```python
from build123d import *

# Parameters (mm, degrees)
SALIENTE_EXTRUIR1_DEPTH    = 25
CORTAR_EXTRUIR1_DEPTH      = 49.94129136
CORTAR_EXTRUIR1_DEPTH_BACK = 49.94129136
CROQUIS2_R                 = 8.375
SALIENTE_EXTRUIR2_DEPTH    = 3
SALIENTE_EXTRUIR3_DEPTH    = 3
CROQUIS5_R                 = 8.375
CORTAR_EXTRUIR2_DEPTH      = 83.95179323
CHAFL_N1_SIZE              = 10
CHAFL_N1_SIZE2             = 24.750868534
CROQUIS6_R                 = 1.625
SALIENTE_EXTRUIR4_DEPTH    = 3
CHAFL_N2_SIZE              = 3


with BuildPart() as part:
    # Croquis1 → Saliente-Extruir1 (new body)
    with BuildSketch(Plane(origin=(0, 0, 0), x_dir=(1, 0, 0), z_dir=(0, 1, 0))):
        Polygon((-26.5, 0), (-26.5, -30), (-29.5, -30), (-29.5, 3), (29.5, 3), (29.5, -30), (26.5, -30), (26.5, 0), align=None)
    extrude(amount=SALIENTE_EXTRUIR1_DEPTH)

    # Croquis2 → Cortar-Extruir1 (cut, two sides: drawn at the far end of the back side and taken through both)
    with BuildSketch(Plane.XY.offset(-CORTAR_EXTRUIR1_DEPTH_BACK)):
        with Locations((-12.925, 12.5)):
            Circle(CROQUIS2_R)
        with Locations(Location((12.925, 12.5, 0), (0, 0, 180))):
            Circle(CROQUIS2_R)
    extrude(amount=CORTAR_EXTRUIR1_DEPTH + CORTAR_EXTRUIR1_DEPTH_BACK, mode=Mode.SUBTRACT)

    # Croquis3 → Saliente-Extruir2 (add)
    with BuildSketch(Plane.ZY.offset(-26.5)):
        Polygon((0, 25), (30, 25), (30, 50), (0, 50), (-3, 50), (-3, 25), align=None)
    extrude(amount=-SALIENTE_EXTRUIR2_DEPTH)

    # Croquis4 → Saliente-Extruir3 (add)
    with BuildSketch(Plane.ZY.offset(29.5)):
        Polygon((0, 25), (30, 25), (30, 50), (0, 50), (-3, 50), (-3, 25), align=None)
    extrude(amount=-SALIENTE_EXTRUIR3_DEPTH)

    # Croquis5 → Cortar-Extruir2 (cut, through all)
    with BuildSketch(Plane.ZY.offset(29.5)):
        with Locations((17.5, 37.925)):
            Circle(CROQUIS5_R)
        with Locations((17.5, 12.075)):
            Circle(CROQUIS5_R)
    extrude(amount=-CORTAR_EXTRUIR2_DEPTH, mode=Mode.SUBTRACT)

    # Chaflán1
    chafl_n1_edges = [part.edges().sort_by_distance(p)[0] for p in [
        (26.5, 25, -1.5),
        (-26.5, 25, -1.5),
    ]]
    chafl_n1_side = [part.faces().sort_by_distance(p)[0] for p in [
        (0, 25, -1.5),
    ]]
    chamfer(chafl_n1_edges, length=CHAFL_N1_SIZE, length2=CHAFL_N1_SIZE2, reference=chafl_n1_side[0])

    # Croquis6 → Saliente-Extruir4 (add)
    # profile 1 of 2: a face of its own
    with BuildSketch(Plane.XY):
        Polygon((-29.5, 0), (-17.5, 0), (-12.5, 0), (-17.5, -5.001983983), (-17.5, -12), (-29.5, -12), align=None)
        with Locations((-23.5, -5.75)):
            Circle(CROQUIS6_R, mode=Mode.SUBTRACT)
    # profile 2 of 2: a face of its own
    with BuildSketch(Plane.XY):
        Polygon((12.5, 0), (17.5, 0), (29.5, 0), (29.5, -12), (17.5, -12), (17.5, -5.001983983), align=None)
        with Locations(Location((23.5, -5.75, 0), (0, 0, 180))):
            Circle(CROQUIS6_R, mode=Mode.SUBTRACT)
    extrude(amount=-SALIENTE_EXTRUIR4_DEPTH)

    # Chaflán2
    chafl_n2_edges = [part.edges().sort_by_distance(p)[0] for p in [
        (-29.5, -12, -1.5),
        (-17.5, -12, -1.5),
        (29.5, -12, -1.5),
        (17.5, -12, -1.5),
    ]]
    chamfer(chafl_n2_edges, length=CHAFL_N2_SIZE)


solid = part.part
```
Geometry check sheet. Reference: the model listing, model coordinates, mm. A direction names the side the tool comes from. Give positions to 0.01 mm unless a question says otherwise; leave off trailing zeros. Write each loop counter-clockwise with the first axis right and the second up, starting at its lowest first coordinate (ties: lowest second). Pieces come first, ordered by that corner, then holes.
1) Section check D-D, the plane z = 17.5. Record the boundary of the cut face in (x, y), and give its area (3 significant figures).
2) Release check for a two-part mould opening along Y. For faces 3 (the flat face through (-19, -10.5, -1.5)), 4 (the flat face through (26.5, 25, 13)), 5 (the cylindrical face through (-28.02, 3.9, 15.68)) record: pulls with the +Y half, pulls with the -Y half, needs draft (parallel to the pull), parting line crosses it, or undercut.
3) Section check A-A, the plane y = -5.75. Record the boundary of the cut face in (x, z) (3 decimals).
4) Access from +Z, -Z, +X, -X, +Y, -Y to the whole of each face (thin tool, end or side, straight path). Record for faces 1 (the flat face through (0, 0, -2)), 2 (the flat face through (-28, 25, 30)).
5) Gauge pin test, flat ends, axial feed: pin 1 (15 mm diameter, centred on y = 37.925, z = 17.5, fed in from -X); pin 2 (1.5 mm diameter, centred on x = -28.5, z = 9, fed in from -Y); pin 3 (19.5 mm diameter, centred on x = 12.925, y = 12.5, fed in from -Z); pin 4 (3.5 mm diameter, centred on x = 0, z = -1, fed in from +Y). Record the tip position at first contact, or that the pin passes through.
6) Section check B-B, the plane z = 3. Record the boundary of the cut face in (x, y).
7) Material ranges on L1, parallel to Y at x = 27, z = 17; L2, parallel to X at y = 27, z = 18; L3, parallel to Y at x = -27, z = 10.5, recorded low to high.
8) Section check C-C, the plane x = 23.5. Record the boundary of the cut face in (y, z) (3 decimals).
Computed:
1. outline: (-29.5, 0) - (-26.5, 0) - (-26.5, 3.7) - (-29.5, 3.7) - close; (-29.5, 20.45) - (-26.5, 20.45) - (-26.5, 29.55) - (-29.5, 29.55) - close; (-29.5, 46.3) - (-26.5, 46.3) - (-26.5, 50) - (-29.5, 50) - close; (26.5, 0) - (29.5, 0) - (29.5, 3.7) - (26.5, 3.7) - close; (26.5, 20.45) - (29.5, 20.45) - (29.5, 29.55) - (26.5, 29.55) - close; (26.5, 46.3) - (29.5, 46.3) - (29.5, 50) - (26.5, 50) - close
1. area: 99.0 mm2
2. face 3: pulls with the -Y half
2. face 4: needs draft
2. face 5: undercut
3. outline: (-29.5, -3) - (-25.125, -3) - (-25.125, 0) - (-29.5, 0) - close; (-21.875, -3) - (-17.5, -3) - (-17.5, 0) - (-21.875, 0) - close; (17.5, -3) - (21.875, -3) - (21.875, 0) - (17.5, 0) - close; (25.125, -3) - (29.5, -3) - (29.5, 0) - (25.125, 0) - close
4. face 1: +Z, -Z, -Y
4. face 2: +Z, +X, -X, +Y, -Y
5. pin 1: passes through
5. pin 2: stops at y = 0
5. pin 3: stops at z = -3
5. pin 4: stops at y = 25
6. outline: (-29.5, 0) - (-26.5, 0) - (-26.5, 50) - (-29.5, 50) - close; (26.5, 0) - (29.5, 0) - (29.5, 50) - (26.5, 50) - close
7. L1: y = 0 to 3.71, 20.44 to 29.56, 46.29 to 50
7. L2: x = -29.5 to -26.5, 26.5 to 29.5
7. L3: y = 0 to 7.48, 16.67 to 33.33, 42.52 to 50
8. outline: (-12, -3) - (-7.375, -3) - (-7.375, 0) - (-12, 0) - close; (-4.125, -3) - (42.326, -3) - (42.326, 0) - (-4.125, 0) - close
